Drawing for the job (mm, zero at the part's lowest x, y, z). Round coordinates to 2 decimals unless told otherwise and drop trailing zeros. Order: outer loops, then holes, each group sorted by start corner. A loop starts at its lowest first (then second) coordinate and runs counter-clockwise, first axis right, second up. Notation, with made-up numbers: (2.25, 51.25) -> (33.25, 51.25) arc R30 cw to (33.25, 90.25) -> close; hole circle Ø3 at (15.5, 41). An arc over 180 degrees is marked (long way). Use CSV: the item, a comma, the result in double quotes.
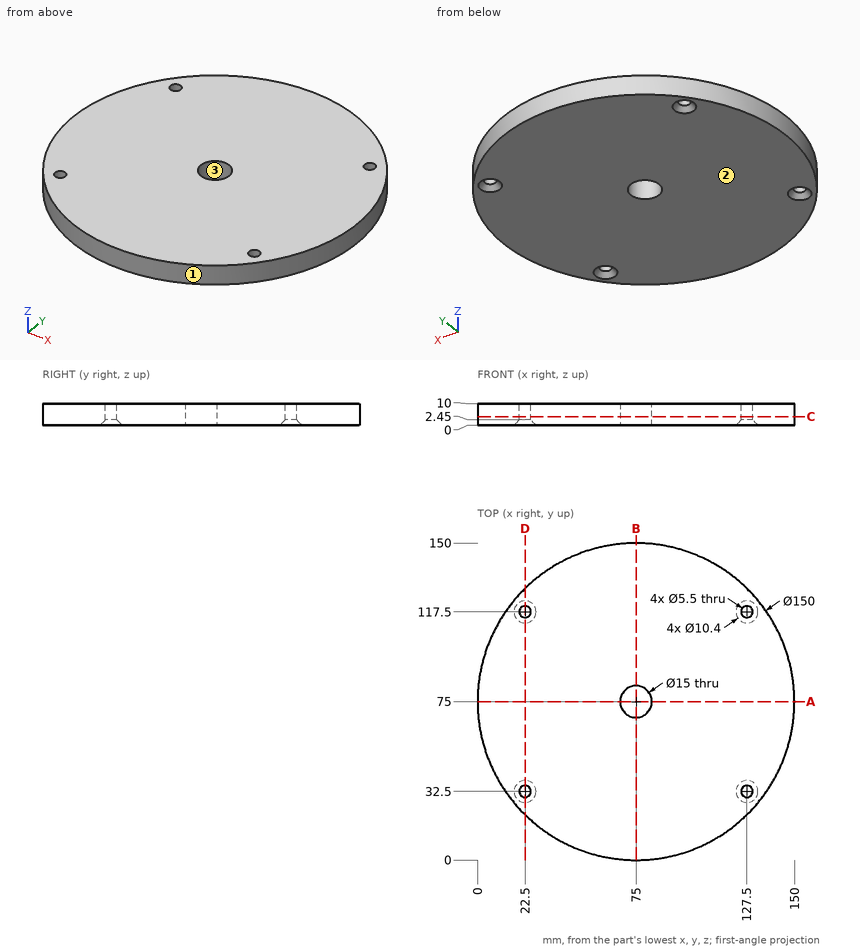
Q1. Cut at C-C (z = 4). Give the cut face in (x, y), plus the area to 3 significant figures.
From the geometry:
outline,"circle Ø150 at (75, 75); hole circle Ø5.5 at (22.5, 32.5); hole circle Ø5.5 at (22.5, 117.5); hole circle Ø15 at (75, 75); hole circle Ø5.5 at (127.5, 32.5); hole circle Ø5.5 at (127.5, 117.5)"
area,"17,400 mm²"
Q2. Cut at A-A (y = 75). Give the cut face in (x, z).
From the geometry:
outline,"(0, 0) -> (67.5, 0) -> (67.5, 10) -> (0, 10) -> close; (82.5, 0) -> (150, 0) -> (150, 10) -> (82.5, 10) -> close"
Q3. Probe line 1 along X through (y, z) = (34.5, 6.5); line 2 along Y through (x, z) = (127.5, 4.75); line 3 along Y through (x, z) = (21, 2). List the from-to ranges inside material, lowest first.
From the geometry:
line 1,"x = 11.88 to 20.61, 24.39 to 125.61, 129.39 to 138.12"
line 2,"y = 21.44 to 29.75, 35.25 to 114.75, 120.25 to 128.56"
line 3,"y = 22.95 to 29.67, 35.33 to 114.67, 120.33 to 127.05"
Q4. Pin check, flat tips, straight feed: pin 1 (7 mm diameter, centred on x = 22.5, y = 117.5, fed in from -Z); pin 2 (6.5 mm diameter, centred on x = 22.5, y = 32.5, fed in from -Z); pin 3 (5 mm diameter, centred on x = 45.5, z = 3, fed in from -Y); pin 4 (9 mm diameter, centred on x = 127.5, y = 117.5, fed in from +Z). Stop position of each tip, or through.
From the geometry:
pin 1,"stops at z = 1.7"
pin 2,"stops at z = 1.95"
pin 3,"stops at y = 5.03"
pin 4,"stops at z = 10"
Q5. Cut at D-D (x = 22.5). Give the cut face in (y, z), plus the area to 3 significant figures.
From the geometry:
outline,"(21.44, 0) -> (27.3, 0) -> (29.75, 2.45) -> (29.75, 10) -> (21.44, 10) -> close; (35.25, 2.45) -> (37.7, 0) -> (112.3, 0) -> (114.75, 2.45) -> (114.75, 10) -> (35.25, 10) -> close; (120.25, 2.45) -> (122.7, 0) -> (128.56, 0) -> (128.56, 10) -> (120.25, 10) -> close"
area,"949 mm²"
Q6. Mould opens along Y. For the marked faces 1, 2 and 3 say: +Y half, -Y half, draft (parallel to the pull), parting line (faces both ways), or undercut.
From the geometry:
face 1,"parting line"
face 2,"draft"
face 3,"undercut"
